Part print with two shaded views. Sizes in mm from the minimum x, y, z corner. A direction names the side the tool comes from. Give positions to 0.01 mm unless a question says otherwise; leave off trailing zeros. Write each loop counter-clockwise with the first axis right and the second up, starting at its lowest first coordinate (ties: lowest second). Pieces come first, ordered by that corner, then holes.
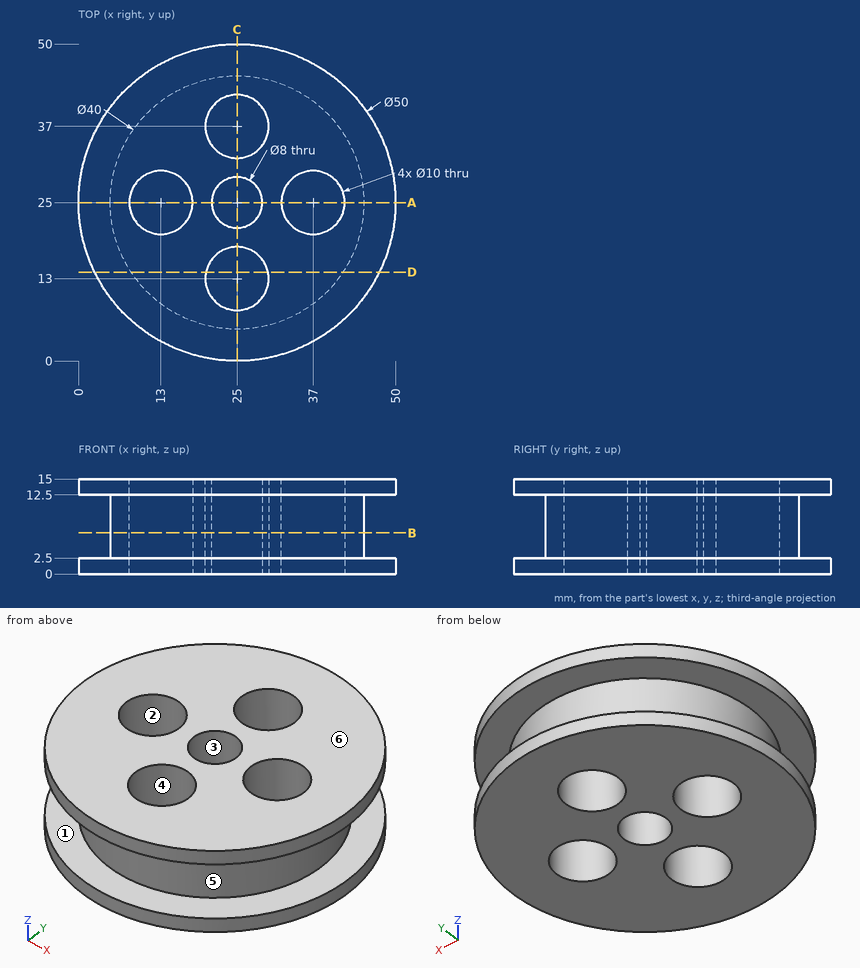
1) Drill centre lines: L1, parallel to Y at x = 40, z = 1.25; L2, parallel to Z at x = 10, y = 44; L3, parallel to X at y = 26, z = 8. Where is each one in solid material? Low to high.
Check result:
L1: y = 5 to 21, 29 to 45
L2: z = 0 to 2.5, 12.5 to 15
L3: x = 5.03 to 8.1, 17.9 to 21.13, 28.87 to 32.1, 41.9 to 44.97
2) Flat gauge pins, fed straight in: P1, Ø2, axis at x = 23, z = 8, coming from the -Y side (3 decimals); P2, Ø1.5, axis at x = 20.5, z = 2, coming from the -Y side; P3, Ø2, axis at x = 35.5, z = 4, coming from the +Y side. Where does each tip first touch, or does it go through?
Check result:
P1: stops at y = 5.025
P2: stops at y = 0.28
P3: stops at y = 42.6
3) Mould opens along X. For the marked faces 3, 4, 5 and 6 say: +X half, -X half, draft (parallel to the pull), parting line (faces both ways), or undercut.
Check result:
face 3: undercut
face 4: undercut
face 5: parting line
face 6: draft
4) Saw through at D-D (y = 14). Write the cut outline in (x, z), and give its area (3 significant figures).
Check result:
outline: (2.55, 0) - (20.1, 0) - (20.1, 15) - (2.55, 15) - (2.55, 12.5) - (8.3, 12.5) - (8.3, 2.5) - (2.55, 2.5) - close; (29.9, 0) - (47.45, 0) - (47.45, 2.5) - (41.7, 2.5) - (41.7, 12.5) - (47.45, 12.5) - (47.45, 15) - (29.9, 15) - close
area: 412 mm2
5) Saw through at B-B (z = 6.5). Write the cut outline in (x, y).
Check result:
outline: circle Ø40 at (25, 25); hole circle Ø10 at (13, 25); hole circle Ø10 at (25, 13); hole circle Ø10 at (25, 37); hole circle Ø8 at (25, 25); hole circle Ø10 at (37, 25)
6) Saw through at A-A (y = 25). Write the cut outline in (x, z).
Check result:
outline: (0, 0) - (8, 0) - (8, 15) - (0, 15) - (0, 12.5) - (5, 12.5) - (5, 2.5) - (0, 2.5) - close; (18, 0) - (21, 0) - (21, 15) - (18, 15) - close; (29, 0) - (32, 0) - (32, 15) - (29, 15) - close; (42, 0) - (50, 0) - (50, 2.5) - (45, 2.5) - (45, 12.5) - (50, 12.5) - (50, 15) - (42, 15) - close
7) 3-axis set-ups, long thin cutter, end or side, ignore diameter. For the marked faces 1 and 2: which of +Z, -Z, +X, -X, +Y, -Y reach the whole face in a straight line?
Check result:
face 1: none
face 2: +Z, -Z
